Design review of the part built by this model. Coordinates are the model's own, in mm. Face numbers are marked on the shaded views. A direction names the side the tool comes from. Give positions to 0.01 mm unless a question says otherwise; leave off trailing zeros. Write each loop counter-clockwise with the first axis right and the second up, starting at its lowest first coordinate (ties: lowest second). Pieces come first, ordered by that corner, then holes. Notation, with made-up numbers: M 73.25,63 L 121.25,63 A20 ccw 121.25,69 Z; hole C -1.75,30.5 d5. An arc over 180 degrees is marked long. Write each question's results on one line, items separated by ' | '. Start each with the question number.
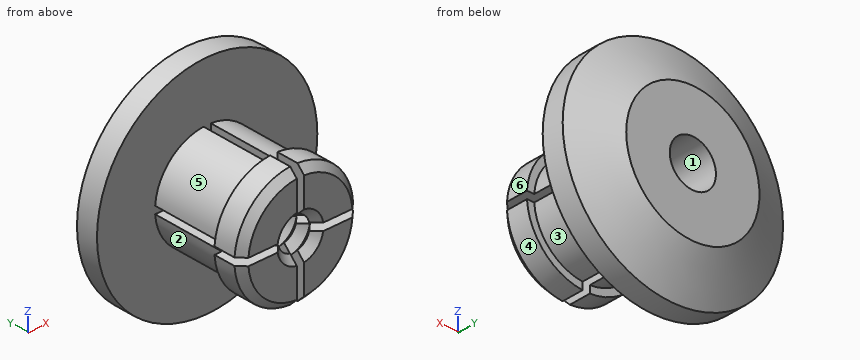
from build123d import *

# Parameters (mm, degrees)
ENL_V_MAT_EXTRU_2_DEPTH = 7


with BuildPart() as part:
    # Esquisse1 → Révolution1 (revolve)
    with BuildSketch(Plane.XY):
        Polygon((1.59, -0.870821866), (4.59, -0.870821866), (7.59, -2.370821866), (7.59, -3.870821866), (3.59, -3.870821866), (3.59, -8.870821866), (4.09, -8.870821866), (4.09, -10.370821866), (3.59, -10.870821866), (1.59, -10.870821866), (1.09, -10.370821866), (1.59, -9.870821866), (1.09, -9.370821866), (1.59, -8.870821866), (1.09, -8.370821866), (1.59, -7.870821866), align=None)
    revolve(axis=Axis((0, 0, 0), (0, 1, 0)))

    # Esquisse4 → Enlèv. mat.-Extru.2 (cut)
    with BuildSketch(Plane.XZ.offset(10.870821866)):
        Polygon((-0.25, 0.25), (-6.93889881, 0.25), (-6.93889881, -0.25), (-0.25, -0.25), (-0.25, -5.58524478), (0.25, -5.58524478), (0.25, -0.25), (11.352493463, -0.25), (11.352493463, 0.25), (0.25, 0.25), (0.25, 5.858250635), (-0.25, 5.858250635), align=None)
    extrude(amount=-ENL_V_MAT_EXTRU_2_DEPTH, mode=Mode.SUBTRACT)


solid = part.part
Q1. For pin 1 Ø0.9 at (y, z) = (-7.5, 3) entering from +X; pin 2 Ø2.5 at (y, z) = (-8.5, 3) entering from -X; pin 3 Ø1.5 at (y, z) = (-7, -2) entering from +X; pin 4 Ø1 at (x, y) = (-4.5, -4.5) entering from +Z, all flat-tipped, find the tip position at first contact; note any pin that passes through.
Q2. We need section B-B on z = 0. Write out the cut boundary in (x, y), and give its area (3 significant figures).
Q3. The part is to be moulded in two halves that separate along X. For the marked faces 1, 2 and 3, say which applies: pulls with the +X half, pulls with the -X half, needs draft (parallel to the pull), parting line crosses it, or undercut.
Q4. We need section D-D on y = -3.5. Write out the cut boundary in (x, z), and give its area (3 significant figures).
Q5. We need section C-C on y = -5. Write out the cut boundary in (x, z).
Q6. For the marked faces 4, 5 and 6, list the 3-axis set-ups (+Z, -Z, +X, -X, +Y, -Y) from which the entire face can be reached by the end or side of a thin tool; tool diameter is ignored.
Q7. Wall thickness on line 1 along X through (y, z) = (-3.25, 0); line 2 along Y through (x, z) = (-2.75, -3.25); line 3 along Z through (x, y) = (-3, -6): over which ranges is each line inside the solid? List them lowest first. Write a range as from..to.
Q8. We need section A-A on x = 0. Write out the cut boundary in (y, z), and give its area (3 significant figures).
Answer sheet:
1) pin 1: x = 2.53 | pin 2: x = -3.67 | pin 3: x = 3.37 | pin 4: through
2) outline: M -7.59,-3.87 L -1.59,-3.87 L -1.59,-0.87 L -4.59,-0.87 L -7.59,-2.37 Z; M 1.59,-3.87 L 7.59,-3.87 L 7.59,-2.37 L 4.59,-0.87 L 1.59,-0.87 Z | area: 31.5 mm^2
3) face 1: undercut | face 2: pulls with the -X half | face 3: pulls with the +X half
4) outline: C 0,0 d15.18; hole C 0,0 d3.18 | area: 173 mm^2
5) outline: M -3.58,-0.25 A3.59 ccw -0.25,-3.58 L -0.25,-1.57 A1.59 cw -1.57,-0.25 Z; M -3.58,0.25 L -1.57,0.25 A1.59 cw -0.25,1.57 L -0.25,3.58 A3.59 ccw Z; M 0.25,-3.58 A3.59 ccw 3.58,-0.25 L 1.57,-0.25 A1.59 cw 0.25,-1.57 Z; M 0.25,1.57 A1.59 cw 1.57,0.25 L 3.58,0.25 A3.59 ccw 0.25,3.58 Z
6) face 4: -Z, +X, -Y | face 5: +Z, -X | face 6: +Z, +X, -Y
7) line 1: -7.59..-1.59, 1.59..7.59 | line 2: -3.87..-0.87 | line 3: -1.97..-0.25, 0.25..1.97
8) outline: M -3.87,-7.59 L -2.37,-7.59 L -0.87,-4.59 L -0.87,-1.59 L -3.87,-1.59 Z; M -3.87,1.59 L -0.87,1.59 L -0.87,4.59 L -2.37,7.59 L -3.87,7.59 Z | area: 31.5 mm^2
